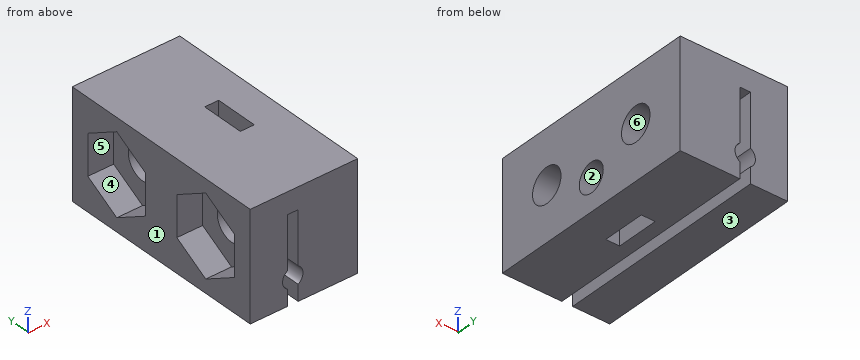
from build123d import *

# Parameters (mm, degrees)
BOX_W           = 10
BOX_H           = 20
BOX_DEPTH       = 10
POCKET_DEPTH    = 20.001
POCKET001_DEPTH = 2.4
SKETCH002_R     = 1.6
POCKET002_DEPTH = 10.001
SKETCH003_W     = 1.3
SKETCH003_H     = 4
POCKET003_DEPTH = 10.001
SKETCH004_R     = 1.35
POCKET004_DEPTH = 3


with BuildPart() as part:
    # Box → Box (new body)
    with BuildSketch(Plane.XY):
        with Locations((5, 10)):
            Rectangle(BOX_W, BOX_H)
    extrude(amount=BOX_DEPTH)

    # Sketch → Pocket (cut, through all)
    with BuildSketch(Plane.XZ):
        with BuildLine():
            Line((3.458295, 0), (3.458295, 1.492225))
            ThreePointArc((3.458295, 3.107775), (3.008295, 2.3), (3.458295, 1.492225))
            Line((3.458295, 3.107775), (3.458295, 8))
            Line((3.458295, 8), (4.458295, 8))
            Line((4.458295, 8), (4.458295, 3.107775))
            ThreePointArc((4.458295, 1.492225), (4.908295, 2.3), (4.458295, 3.107775))
            Line((4.458295, 1.492225), (4.458295, 0))
            Line((3.458295, 0), (4.458295, 0))
        make_face()
    extrude(amount=-POCKET_DEPTH, mode=Mode.SUBTRACT)

    # Sketch001 → Pocket001 (cut)
    with BuildSketch(Plane(origin=(0, 0, 0), x_dir=(0, -1, 0), z_dir=(-1, 0, 0))):
        Polygon((-8.25, 6.876388), (-8.25, 3.123612), (-5, 1.247223), (-1.75, 3.123612), (-1.75, 6.876388), (-5, 8.752777), align=None)
        Polygon((-18.25, 6.876388), (-18.25, 3.123612), (-15, 1.247223), (-11.75, 3.123612), (-11.75, 6.876388), (-15, 8.752777), align=None)
    extrude(amount=-POCKET001_DEPTH, mode=Mode.SUBTRACT)

    # Sketch002 → Pocket002 (cut, through all)
    with BuildSketch(Plane.YZ.offset(10)):
        with Locations((5, 5)):
            Circle(SKETCH002_R)
        with Locations((15, 5)):
            Circle(SKETCH002_R)
    extrude(amount=-POCKET002_DEPTH, mode=Mode.SUBTRACT)

    # Sketch003 → Pocket003 (cut, through all)
    with BuildSketch(Plane.XY.offset(10)):
        with Locations((6.35, 10)):
            Rectangle(SKETCH003_W, SKETCH003_H)
    extrude(amount=-POCKET003_DEPTH, mode=Mode.SUBTRACT)

    # Sketch004 → Pocket004 (cut)
    with BuildSketch(Plane.YZ.offset(10)):
        with Locations((10, 3)):
            Circle(SKETCH004_R)
    extrude(amount=-POCKET004_DEPTH, mode=Mode.SUBTRACT)


solid = part.part
CAD build for the part. Positions are in the model's coordinates, mm. Face numbers are marked on the shaded views. A direction names the side the tool comes from. Round coordinates to 2 decimals unless told otherwise and drop trailing zeros. Write each loop counter-clockwise with the first axis right and the second up, starting at its lowest first coordinate (ties: lowest second). Pieces come first, ordered by that corner, then holes. Notation, with made-up numbers: M 10.5,-18 L 31.5,-18 A19 ccw 31.5,7 Z; hole C 27.25,22.5 d7. An arc over 180 degrees is marked long. Put each result on its own line as item: value. Start each with the question number.
1) Pull direction Z, two halves, no side cores. Call the marked faces 1, 2, 3 and 4: pulls with the +Z half, pulls with the -Z half, needs draft (parallel to the pull), parting line crosses it, or undercut.
2) Saw through at C-C, the plane x = 6. Write the cut outline in (y, z).
3) Drill centre lines: probe 1 along X at (y, z) = (6, 7.75); probe 2 along Z at (x, y) = (7.85, 15); probe 3 along Y at (x, z) = (3, 6). Where is each one in solid material? Low to high. Write a range as [from, to].
4) Saw through at A-A, the plane z = 1. Write the cut outline in (x, y), and give its area (3 significant figures).
5) Pin check, flat tips, straight feed: pin 1 Ø2.5 at (y, z) = (10, 3) entering from +X; pin 2 Ø2 at (y, z) = (6.5, 5) entering from -X; pin 3 Ø0.8 at (x, y) = (4, 12) entering from -Z; pin 4 Ø2.5 at (y, z) = (5, 5) entering from -X. Stop position of each tip, or through.
6) Saw through at B-B, the plane y = 10. Write the cut outline in (x, z), and give its area (3 significant figures).
7) Saw through at D-D, the plane z = 8.5. Write the cut outline in (x, y).
8) 3-axis set-ups, long thin cutter, end or side, ignore diameter. For the marked faces 5 and 6: which of +Z, -Z, +X, -X, +Y, -Y reach the whole face in a straight line?
Resolved:
1. face 1: needs draft
1. face 2: undercut
1. face 3: pulls with the -Z half
1. face 4: undercut
2. outline: M 0,0 L 8,0 L 8,10 L 0,10 Z; M 12,0 L 20,0 L 20,10 L 12,10 Z; hole C 5,5 d3.2; hole C 15,5 d3.2
3. probe 1: [2.4, 3.46], [4.46, 10]
3. probe 2: [0, 3.4], [6.6, 10]
3. probe 3: [0, 3.75], [6.25, 13.75], [16.25, 20]
4. outline: M 0,0 L 3.46,0 L 3.46,20 L 0,20 Z; M 4.46,0 L 10,0 L 10,20 L 4.46,20 Z; hole M 5.7,8 L 7,8 L 7,12 L 5.7,12 Z
4. area: 175 mm²
5. pin 1: x = 5.7
5. pin 2: x = 2.4
5. pin 3: z = 8
5. pin 4: through
6. outline: M 0,0 L 3.46,0 L 3.46,1.49 A0.95 cw 3.46,3.11 L 3.46,8 L 4.46,8 L 4.46,3.11 A0.95 cw 4.46,1.49 L 4.46,0 L 5.7,0 L 5.7,10 L 0,10 Z; M 7,0 L 10,0 L 10,1.65 L 7,1.65 Z; M 7,4.35 L 10,4.35 L 10,10 L 7,10 Z
6. area: 69.9 mm²
7. outline: M 0,0 L 10,0 L 10,20 L 0,20 L 0,15.44 L 2.4,15.44 L 2.4,14.56 L 0,14.56 L 0,5.44 L 2.4,5.44 L 2.4,4.56 L 0,4.56 Z; hole M 5.7,8 L 7,8 L 7,12 L 5.7,12 Z
8. face 5: -X
8. face 6: +X, -X
